Here's how the part is built. I have some questions about the finished solid (model axes, mm). A direction names the side the tool comes from. Round coordinates to 2 decimals unless told otherwise and drop trailing zeros. Order: outer loops, then holes, each group sorted by start corner. A loop starts at its lowest first (then second) coordinate and runs counter-clockwise, first axis right, second up. Notation, with made-up numbers: (-13.5, -35.75) -> (36.5, -35.75) arc R19 cw to (36.5, -8.75) -> close; hole circle Ø2 at (23, -23). An arc over 180 degrees is marked (long way). Answer in a Markdown table with one row per item.
```python
from build123d import *

# Parameters (mm, degrees)
SKETCH_R     = 38.5
PAD_DEPTH    = 40
SKETCH001_R  = 36
POCKET_DEPTH = 37
FILLET_R     = 1
FILLET001_R  = 2
FILLET002_R  = 1


with BuildPart() as part:
    # Sketch → Pad (new body)
    with BuildSketch(Plane.XY):
        Circle(SKETCH_R)
    extrude(amount=PAD_DEPTH)

    # Sketch001 (on Face3 of Pad) → Pocket (cut)
    with BuildSketch(Plane.XY.offset(40)):
        Circle(SKETCH001_R)
    extrude(amount=-POCKET_DEPTH, mode=Mode.SUBTRACT)

    # Fillet
    fillet_edges = [part.edges().sort_by_distance(p)[0] for p in [
        (-38.5, 0, 40),
        (-36, 0, 40),
    ]]
    fillet(fillet_edges, radius=FILLET_R)

    # Fillet001
    fillet001_edges = [part.edges().sort_by_distance(p)[0] for p in [
        (-38.5, 0, 0),
    ]]
    fillet(fillet001_edges, radius=FILLET001_R)

    # Fillet002
    fillet002_edges = [part.edges().sort_by_distance(p)[0] for p in [
        (-36, 0, 3),
    ]]
    fillet(fillet002_edges, radius=FILLET002_R)


solid = part.part
```
1. For pin 1 Ø5 at (x, y) = (-6, 26) entering from +Z; pin 2 Ø3 at (x, z) = (6, 22.5) entering from -Y; pin 3 Ø2 at (x, z) = (-8.5, 10.5) entering from -Y, each with a flat end and sliding along its axis, tell me the tip position at first contact or that it passes through.
Numbers:
| item | result |
|---|---|
| pin 1 | stops at z = 3 |
| pin 2 | stops at y = -38.24 |
| pin 3 | stops at y = -37.76 |
2. For faces 1 (the face through (0, 0, 3)), 2 (the face through (-1, 1, 0)), which set-ups out of +Z, -Z, +X, -X, +Y, -Y let a thin tool reach every point of the face, with its end or its side?
Numbers:
| item | result |
|---|---|
| face 1 | +Z |
| face 2 | -Z, +X, -X, +Y, -Y |
3. Suppose I cut it at C-C on z = 31. Write out the boundary of the cut face in (x, y).
Numbers:
| item | result |
|---|---|
| outline | circle Ø77 at (0, 0); hole circle Ø72 at (0, 0) |
4. Suppose I cut it at A-A on x = 0. Write out the boundary of the cut face in (y, z).
Numbers:
| item | result |
|---|---|
| outline | (-38.5, 2) arc R2 ccw to (-36.5, 0) -> (36.5, 0) arc R2 ccw to (38.5, 2) -> (38.5, 39) arc R1 ccw to (37.5, 40) -> (37, 40) arc R1 ccw to (36, 39) -> (36, 4) arc R1 cw to (35, 3) -> (-35, 3) arc R1 cw to (-36, 4) -> (-36, 39) arc R1 ccw to (-37, 40) -> (-37.5, 40) arc R1 ccw to (-38.5, 39) -> close |
5. We'd pull the mould along X, two halves only. Please class faces 3 (the face through (-30.55, -23.43, 20.24)), 4 (the face through (-4.686, 35.694, 21.745)), 5 (the face through (33.2, 16.8, 40)): released by +X, released by -X, zero draft, split by the parting line, or undercut.
Numbers:
| item | result |
|---|---|
| face 3 | split by the parting line |
| face 4 | undercut |
| face 5 | zero draft |
6. Please list where these lines run through material, in increasing order: line 1 along Y through (x, z) = (0, 18); line 2 along Z through (x, y) = (-33, -1); line 3 along Y through (x, z) = (11, 17).
Numbers:
| item | result |
|---|---|
| line 1 | y = -38.5 to -36, 36 to 38.5 |
| line 2 | z = 0 to 3 |
| line 3 | y = -36.9 to -34.28, 34.28 to 36.9 |
